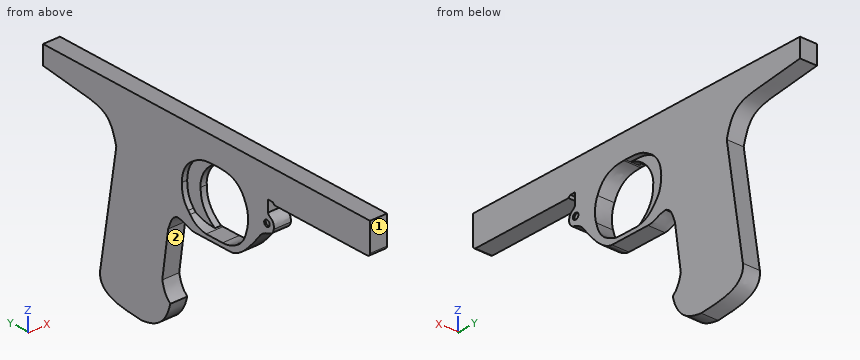
```python
from build123d import *

# Parameters (mm, degrees)
F0_W     = 69.4504092897
F0_H     = 8
F1_DEPTH = 11
F2_DEPTH = 7.5
F3_DEPTH = 3.5
F4_R     = 2
F5_DEPTH = 1
F6_R     = 2
F7_DEPTH = 1
F8_R     = 2


with BuildPart() as f1:
    # F0 (on Right) → F1 (new body)
    with BuildSketch(Plane.YZ):
        Polygon((125.9671086108, -218), (0, -218), (0, -230), (119.9886596101, -230), (125.9671086108, -230), align=None)
        Polygon((0, -230), (0, -218), (-112.0328913892, -218), (-112.0328913892, -230), (-42.5824820995, -230), align=None)
        with BuildLine():
            Line((119.9886596101, -230), (0, -230))
            Line((0, -230), (-42.5824820995, -230))
            Line((-42.5824820995, -230), (-42.5824820995, -238))
            Line((-42.5824820995, -238), (-41.2151366472, -236.7386668921))
            Line((-41.2151366472, -236.7386668921), (-37.7865731716, -236.7386668921))
            Line((-37.7865731716, -236.7386668921), (-37.7865731716, -243.9223229885))
            add(Edge.make_bspline(
                [(-42.0314595103, -251.4325082302), (-42.5212569535, -245.88149786), (-38.4396314621, -246.6978281736), (-37.7865731716, -243.9223229885)],
                knots=[0, 0, 0, 0, 8.62681531, 8.62681531, 8.62681531, 8.62681531], degree=3))
            add(Edge.make_bspline(
                [(-32.398827374, -258.4528923035), (-36.9702465832, -254.0447413921), (-40.8886037767, -256.6569745541), (-42.0314595103, -251.4325082302)],
                knots=[0, 0, 0, 0, 11.919454451, 11.919454451, 11.919454451, 11.919454451], degree=3))
            add(Edge.make_bspline(
                [(-10.8478534967, -276.8577933311), (-18.0315114558, -276.4120399952), (-25.3784339875, -267.5957381725), (-32.398827374, -258.4528923035)],
                knots=[0, 0, 0, 0, 28.3405161721, 28.3405161721, 28.3405161721, 28.3405161721], degree=3))
            Line((-10.8478534967, -276.8577933311), (15.3035437688, -276.8577933311))
            add(Edge.make_bspline(
                [(28.3146612346, -273.5956013203), (22.7218363434, -273.8401889801), (20.3328952193, -276.941627264), (15.3035437688, -276.8577933311)],
                knots=[0, 0, 0, 0, 13.4138389145, 13.4138389145, 13.4138389145, 13.4138389145], degree=3))
            add(Edge.make_bspline(
                [(34.9013535306, -282.8655987978), (33.5207916796, -280.2323997021), (33.0320037901, -274.9298810959), (28.3146612346, -273.5956013203)],
                knots=[0, 0, 0, 0, 11.3717794841, 11.3717794841, 11.3717794841, 11.3717794841], degree=3))
            Line((34.9013535306, -282.8655987978), (30.6285899132, -252.9632747173))
            Line((30.6285899132, -252.9632747173), (72.6285899132, -252.9632747173))
            add(Edge.make_bspline(
                [(125.9671086108, -230), (84.4510868192, -236.0368669033), (78.2147446722, -231.554299593), (72.6285899132, -252.9632747173)],
                knots=[0, 0, 0, 0, 58.0715899782, 58.0715899782, 58.0715899782, 58.0715899782], degree=3))
            Line((125.9671086108, -230), (119.9886596101, -230))
        make_face()
        with BuildLine():
            add(Edge.make_bspline(
                [(-2.2899068426, -233.791783452), (-6.7162262276, -233.9929789305), (-16.5748465806, -233.5905879736), (-21.4035585523, -245.2599704266)],
                knots=[0, 0, 0, 0, 22.2901546464, 22.2901546464, 22.2901546464, 22.2901546464], degree=3))
            add(Edge.make_bspline(
                [(-1.1649398204, -233.7192680463), (-1.5450471165, -233.73570765), (-1.920463643, -233.7595033317), (-2.2899068426, -233.791783452)],
                knots=[0.9357244438, 0.9357244438, 0.9357244438, 0.9357244438, 1, 1, 1, 1], degree=3))
            add(Edge.make_bspline(
                [(18.53771694, -239.1283065081), (12.2761912644, -234.5663458109), (6.8953128785, -233.9907415129), (0.97691075, -233.6266332169), (-1.1649398204, -233.7192680463)],
                knots=[0, 0, 0, 0, 0.5735408235, 0.9357244438, 0.9357244438, 0.9357244438, 0.9357244438], degree=3))
            add(Edge.make_bspline(
                [(24.9781440943, -253.0825734138), (24.7097946703, -247.3577409983), (23.0102371424, -242.7957803011), (18.53771694, -239.1283065081)],
                knots=[0, 0, 0, 0, 15.3688212563, 15.3688212563, 15.3688212563, 15.3688212563], degree=3))
            add(Edge.make_bspline(
                [(20.3267261386, -266.5895819664), (23.9941906184, -262.5643014908), (24.7992426157, -258.628487587), (24.9781440943, -253.0825734138)],
                knots=[0, 0, 0, 0, 14.2854810573, 14.2854810573, 14.2854810573, 14.2854810573], degree=3))
            add(Edge.make_bspline(
                [(18.8836723567, -268.3176113068), (19.3763812768, -267.758725569), (19.8515536715, -267.1799487583), (20.3267261386, -266.5895819664)],
                knots=[12.7076946491, 12.7076946491, 12.7076946491, 12.7076946491, 15.1457642124, 15.1457642124, 15.1457642124, 15.1457642124], degree=3))
            add(Edge.make_bspline(
                [(7.2669684887, -274.2601037025), (13.2710677225, -273.603274134), (16.3155772532, -271.2306329063), (18.8836723567, -268.3176113068)],
                knots=[0, 0, 0, 0, 12.7076946491, 12.7076946491, 12.7076946491, 12.7076946491], degree=3))
            Line((7.2669684887, -274.2601037025), (-4.6425154433, -274.2601037025))
            add(Edge.make_bspline(
                [(-13.254606165, -272.155880928), (-8.8760508224, -274.2601037025), (-7.2994241491, -274.2016911507), (-4.6425154433, -274.2601037025)],
                knots=[0, 0, 0, 0, 8.8654306203, 8.8654306203, 8.8654306203, 8.8654306203], degree=3))
            add(Edge.make_bspline(
                [(-22.3616603762, -259.9363029003), (-21.093590185, -266.046077013), (-18.2116106153, -269.9655890465), (-13.254606165, -272.155880928)],
                knots=[0, 0, 0, 0, 15.2399646844, 15.2399646844, 15.2399646844, 15.2399646844], degree=3))
            add(Edge.make_bspline(
                [(-21.4035585523, -245.2599704266), (-23.62973243, -249.4458854198), (-23.7450096756, -255.9015154839), (-22.3616603762, -259.9363029003)],
                knots=[0, 0, 0, 0, 14.7075726748, 14.7075726748, 14.7075726748, 14.7075726748], degree=3))
        make_face(mode=Mode.SUBTRACT)
        with Locations((-77.3076867444, -234)):
            Rectangle(F0_W, F0_H)
        with BuildLine():
            Line((84.3787366599, -326.129257679), (72.6285899132, -252.9632747173))
            Line((72.6285899132, -252.9632747173), (30.6285899132, -252.9632747173))
            Line((30.6285899132, -252.9632747173), (34.9013535306, -282.8655987978))
            Line((34.9013535306, -282.8655987978), (39.1741171479, -312.7679228783))
            add(Edge.make_bspline(
                [(39.1741171479, -312.7679228783), (37.5588834286, -320.5303251743), (34.5356166363, -322.179377079), (33.2988277078, -323.5535919666)],
                knots=[0, 0, 0, 0, 12.2820879206, 12.2820879206, 12.2820879206, 12.2820879206], degree=3))
            add(Edge.make_bspline(
                [(33.2988277078, -323.5535919666), (37.0091982186, -338.8073444366), (47.0409430563, -340.4563963413), (54.0494211018, -341.2809073925)],
                knots=[0, 0, 0, 0, 27.2918456396, 27.2918456396, 27.2918456396, 27.2918456396], degree=3))
            add(Edge.make_bspline(
                [(54.0494211018, -341.2809073925), (62.8443732858, -340.3189778328), (86.0685482621, -340.8686518669), (84.3787366599, -326.129257679)],
                knots=[0, 0, 0, 0, 33.9033902621, 33.9033902621, 33.9033902621, 33.9033902621], degree=3))
        make_face()
    extrude(amount=F1_DEPTH)

    # F0 (on Right) → F2 (join)
    with BuildSketch(Plane.YZ):
        with BuildLine():
            add(Edge.make_bspline(
                [(18.53771694, -239.1283065081), (12.2761912644, -234.5663458109), (6.8953128785, -233.9907415129), (0.97691075, -233.6266332169), (-1.1649398204, -233.7192680463)],
                knots=[0, 0, 0, 0, 0.5735408235, 0.9357244438, 0.9357244438, 0.9357244438, 0.9357244438], degree=3))
            add(Edge.make_bspline(
                [(-1.1649398204, -233.7192680463), (12.3649053276, -237.1022552252), (15.8728584647, -248.8357573748), (15.1470759884, -252.9485225677)],
                knots=[0, 0, 0, 0, 25.215988761, 25.215988761, 25.215988761, 25.215988761], degree=3))
            add(Edge.make_bspline(
                [(15.1470759884, -252.9485225677), (15.2591429651, -257.8095793724), (14.3406344578, -265.0264501572), (4.7619077377, -271.3247835636)],
                knots=[0, 0, 0, 0, 21.107787373, 21.107787373, 21.107787373, 21.107787373], degree=3))
            add(Edge.make_bspline(
                [(4.7619077377, -271.3247835636), (7.9766856506, -271.1279392242), (11.5851107985, -271.3903784752), (18.8836723567, -268.3176113068)],
                knots=[0, 0, 0, 0, 14.4383974504, 14.4383974504, 14.4383974504, 14.4383974504], degree=3))
            add(Edge.make_bspline(
                [(18.8836723567, -268.3176113068), (19.3763812768, -267.758725569), (19.8515536715, -267.1799487583), (20.3267261386, -266.5895819664)],
                knots=[12.7076946491, 12.7076946491, 12.7076946491, 12.7076946491, 15.1457642124, 15.1457642124, 15.1457642124, 15.1457642124], degree=3))
            add(Edge.make_bspline(
                [(20.3267261386, -266.5895819664), (23.9941906184, -262.5643014908), (24.7992426157, -258.628487587), (24.9781440943, -253.0825734138)],
                knots=[0, 0, 0, 0, 14.2854810573, 14.2854810573, 14.2854810573, 14.2854810573], degree=3))
            add(Edge.make_bspline(
                [(24.9781440943, -253.0825734138), (24.7097946703, -247.3577409983), (23.0102371424, -242.7957803011), (18.53771694, -239.1283065081)],
                knots=[0, 0, 0, 0, 15.3688212563, 15.3688212563, 15.3688212563, 15.3688212563], degree=3))
        make_face()
    extrude(amount=F2_DEPTH)

    # F0 (on Right) → F3 (cut)
    with BuildSketch(Plane.YZ):
        with BuildLine():
            add(Edge.make_bspline(
                [(18.53771694, -239.1283065081), (12.2761912644, -234.5663458109), (6.8953128785, -233.9907415129), (0.97691075, -233.6266332169), (-1.1649398204, -233.7192680463)],
                knots=[0, 0, 0, 0, 0.5735408235, 0.9357244438, 0.9357244438, 0.9357244438, 0.9357244438], degree=3))
            add(Edge.make_bspline(
                [(-1.1649398204, -233.7192680463), (12.3649053276, -237.1022552252), (15.8728584647, -248.8357573748), (15.1470759884, -252.9485225677)],
                knots=[0, 0, 0, 0, 25.215988761, 25.215988761, 25.215988761, 25.215988761], degree=3))
            add(Edge.make_bspline(
                [(15.1470759884, -252.9485225677), (15.2591429651, -257.8095793724), (14.3406344578, -265.0264501572), (4.7619077377, -271.3247835636)],
                knots=[0, 0, 0, 0, 21.107787373, 21.107787373, 21.107787373, 21.107787373], degree=3))
            add(Edge.make_bspline(
                [(4.7619077377, -271.3247835636), (7.9766856506, -271.1279392242), (11.5851107985, -271.3903784752), (18.8836723567, -268.3176113068)],
                knots=[0, 0, 0, 0, 14.4383974504, 14.4383974504, 14.4383974504, 14.4383974504], degree=3))
            add(Edge.make_bspline(
                [(18.8836723567, -268.3176113068), (19.3763812768, -267.758725569), (19.8515536715, -267.1799487583), (20.3267261386, -266.5895819664)],
                knots=[12.7076946491, 12.7076946491, 12.7076946491, 12.7076946491, 15.1457642124, 15.1457642124, 15.1457642124, 15.1457642124], degree=3))
            add(Edge.make_bspline(
                [(20.3267261386, -266.5895819664), (23.9941906184, -262.5643014908), (24.7992426157, -258.628487587), (24.9781440943, -253.0825734138)],
                knots=[0, 0, 0, 0, 14.2854810573, 14.2854810573, 14.2854810573, 14.2854810573], degree=3))
            add(Edge.make_bspline(
                [(24.9781440943, -253.0825734138), (24.7097946703, -247.3577409983), (23.0102371424, -242.7957803011), (18.53771694, -239.1283065081)],
                knots=[0, 0, 0, 0, 15.3688212563, 15.3688212563, 15.3688212563, 15.3688212563], degree=3))
        make_face()
    extrude(amount=F3_DEPTH, mode=Mode.SUBTRACT)

    # F4 (on face) → F5 (cut)
    with BuildSketch(Plane.YZ.offset(11)):
        with Locations((-37.3534969985, -250.1350045204)):
            Circle(F4_R)
    extrude(amount=-F5_DEPTH, mode=Mode.SUBTRACT)

    # F6 (on face) → F7 (cut)
    with BuildSketch(Plane.YZ):
        with Locations((-36.9937494397, -250.1918673515)):
            Circle(F6_R)
    extrude(amount=F7_DEPTH, mode=Mode.SUBTRACT)

    # F8
    f8_edges = [f1.edges().sort_by_distance(p)[0] for p in [
        (5.5, -112.032891, -238),
    ]]
    fillet(f8_edges, radius=F8_R)


solid = f1.part
```
CAD build for the part. Positions are in the model's coordinates, mm. Face numbers are marked on the shaded views. Round coordinates to 2 decimals unless told otherwise and drop trailing zeros. Loops run counter-clockwise (first coordinate to the right, second up) from the corner with the lowest first, then second, coordinate; pieces in that order, holes last. Notation, with made-up numbers: M 67,38.25 L 123,38.25 A15 ccw 123,63.25 Z; hole C -22,6.5 d3. An arc over 180 degrees is marked long. Use a Markdown table: item, result. Add a question column.
(1) Drill centre lines: line 1 (Z direction, x = 6.5, y = 6); line 2 (Z direction, x = 7.75, y = -90.5); line 3 (Z direction, x = 3.25, y = 95.5). Where is each one in solid material? Low to high.
(2) Pull direction Z, two halves, no side cores. Call the marked faces 1 and 2: +Z half, -Z half, draft (parallel to the pull), parting line (faces both ways), or undercut.
(3) Cut at A-A (y = -82). Give the cut face in (x, z).
(4) Flat gauge pins, fed straight in: pin 1 (3 mm diameter, centred on y = -37, z = -250.5, fed in from -X); pin 2 (1.7 mm diameter, centred on x = 4.5, y = -39.5, fed in from -Z); pin 3 (6.5 mm diameter, centred on y = -36.99, z = -250.19, fed in from -X); pin 4 (5.5 mm diameter, centred on x = 5.5, y = -84, fed in from -Z). Where does each tip first touch, or does it go through?
(5) Cut at B-B (z = -288). Give the cut face in (x, y), and give its area (3 significant figures).
Geometry says:
| question | item | result |
|---|---|---|
| 1 | line 1 | z = -276.86 to -274.26, -271.26 to -270.47, -236.75 to -218 |
| 1 | line 2 | z = -238 to -218 |
| 1 | line 3 | z = -233.8 to -218 |
| 2 | face 1 | draft |
| 2 | face 2 | undercut |
| 3 | outline | M 0,-238 L 11,-238 L 11,-218 L 0,-218 Z |
| 4 | pin 1 | stops at x = 1 |
| 4 | pin 2 | stops at z = -255.2 |
| 4 | pin 3 | stops at x = 0 |
| 4 | pin 4 | stops at z = -238 |
| 5 | outline | M 0,35.64 L 11,35.64 L 11,78.26 L 0,78.26 Z |
| 5 | area | 469 mm² |
